```python
from build123d import *

# Parameters (mm, degrees)
F0_W     = 50.8
F0_H     = 50.8
F1_DEPTH = 1.5875
F4_R     = 2.54


with BuildPart() as f1:
    # F0 (on Top) → F1 (new body, symmetric)
    with BuildSketch(Plane.XY):
        Rectangle(F0_W, F0_H)
    extrude(amount=F1_DEPTH, both=True)

    # F2 (on Front) → F3 (revolve, cut)
    with BuildSketch(Plane.XZ):
        Polygon((2.5781, 1.5875), (0, 1.5875), (0, -1.5875), (1.6891, -1.5875), (1.6891, 1.0795), (2.5781, 1.0795), align=None)
    revolve(axis=Axis((0, 0, 3.175), (0, 0, 1)), mode=Mode.SUBTRACT)

    # F4
    f4_edges = [f1.edges().sort_by_distance(p)[0] for p in [
        (-25.4, -25.4, 0),
        (25.4, -25.4, 0),
        (25.4, 25.4, 0),
        (-25.4, 25.4, 0),
    ]]
    fillet(f4_edges, radius=F4_R)


solid = f1.part
```
CAD build for the part. Positions are in the model's coordinates, mm. A direction names the side the tool comes from. Round coordinates to 2 decimals unless told otherwise and drop trailing zeros. Order: outer loops, then holes, each group sorted by start corner. A loop starts at its lowest first (then second) coordinate and runs counter-clockwise, first axis right, second up. Notation, with made-up numbers: (28, 52) - (36, 52) arc R12 ccw to (36, 65) - close; hole circle Ø1 at (50, 42.5). An arc over 180 degrees is marked (long way). Answer as CSV lines item,"result". Start each with the question number.
1. Pull direction Y, two halves, no side cores. Call faces 1 (the face through (24.636, -24.676, 0.022)), 2 (the face through (25.4, 0, 0)), 3 (the face through (-2, -1, 1.08)): +Y half, -Y half, draft (parallel to the pull), parting line (faces both ways), or undercut.
2. Saw through at A-A, the plane y = 0. Write the cut outline in (x, z).
3. Drill centre lines: L1, parallel to Y at x = 0, z = -0.8; L2, parallel to Y at x = 0, z = 1.5. Where is each one in solid material? Low to high. Write a range as [from, to].
4. Pin check, flat tips, straight feed: pin 1 (2.5 mm diameter, centred on x = 0, y = 0, fed in from -Z); pin 2 (4 mm diameter, centred on x = -0.5, y = 0, fed in from +Z). Stop position of each tip, or through.
5. Tool access for faces 4 (the face through (5, 0, 1.588)), 5 (the face through (1.39, 2.17, 1.34)): list every direction of +Z, -Z, +X, -X, +Y, -Y with a clear straight run to the whole face (end or side of a thin tool).
Model answer:
1,face 1,"-Y half"
1,face 2,"draft"
1,face 3,"undercut"
2,outline,"(-25.4, -1.59) - (-1.69, -1.59) - (-1.69, 1.08) - (-2.58, 1.08) - (-2.58, 1.59) - (-25.4, 1.59) - close; (1.69, -1.59) - (25.4, -1.59) - (25.4, 1.59) - (2.58, 1.59) - (2.58, 1.08) - (1.69, 1.08) - close"
3,L1,"y = [-25.4, -1.69], [1.69, 25.4]"
3,L2,"y = [-25.4, -2.58], [2.58, 25.4]"
4,pin 1,"passes through"
4,pin 2,"stops at z = 1.08"
5,face 4,"+Z, +X, -X, +Y, -Y"
5,face 5,"+Z"
